Design review of the part built by this model. Coordinates are the model's own, in mm. A direction names the side the tool comes from. Round coordinates to 2 decimals unless told otherwise and drop trailing zeros. Order: outer loops, then holes, each group sorted by start corner. A loop starts at its lowest first (then second) coordinate and runs counter-clockwise, first axis right, second up. Notation, with made-up numbers: (84, 72) - (116, 72) arc R22 ccw to (116, 79) - close; hole circle Ø3 at (36.5, 59.5). An arc over 180 degrees is marked (long way). Use CSV: the item, a comma, the result in double quotes. Start each with the question number.
from build123d import *

# Parameters (mm, degrees)
BASEHEAD_DEPTH = 19.05
HEADFILLET_R   = 1.524


with BuildPart() as part:
    # Sketch1 → BaseHead (new, symmetric)
    with BuildSketch(Plane.XY):
        Polygon((0, -19.05), (0, 19.05), (19.8374, 19.05), (13.495821211, -19.05), align=None)
    extrude(amount=BASEHEAD_DEPTH, both=True)

    # BodySke → Body (revolve)
    with BuildSketch(Plane.XY, mode=Mode.PRIVATE) as body_sk:
        Polygon((0, 0), (0, 12.7), (90.976850605, 12.7), (92.866610605, 10.81024), (92.866610605, 0), align=None)
    revolve(body_sk.sketch.rotate(Axis((0, 0, 0), (1, 0, 0)), 90), axis=Axis((0, 0, 0), (1, 0, 0)))

    # Sketch3 → HeadChamfer (revolve, cut)
    with BuildSketch(Plane(origin=(0, 0, 0), x_dir=(1, 0, 0), z_dir=(0, -0.7071067811865476, 0.7071067811865475))):
        Polygon((0, 19.05), (9.601632975, 39.640768363), (-6.35, 39.640768363), (-6.35, 19.05), align=None)
    revolve(axis=Axis((0, 0, 0), (1, 0, 0)), mode=Mode.SUBTRACT)

    # HeadFillet
    headfillet_edges = [part.edges().sort_by_distance(p)[0] for p in [
        (16.666610593, -7.7e-08, -12.7),
    ]]
    fillet(headfillet_edges, radius=HEADFILLET_R)


solid = part.part
Q1. Tool access review of faces 1 (the cylindrical face through (53.802, -12.592, -1.653)), 2 (the flat face through (10, 0, -19.05)): name each direction out of +Z, -Z, +X, -X, +Y, -Y from which nothing blocks a thin tool from reaching the whole face with its end or side.
Q2. Clearance check with flat-ended pins moving along their axes: pin 1 (1 mm diameter, centred on x = 29, y = 11.5, fed in from -Z); pin 2 (5 mm diameter, centred on x = 65.5, y = -5.5, fed in from +Z); pin 3 (10 mm diameter, centred on x = 69, z = 13, fed in from -Y). State where each tip first meets the part, or that it passes through.
Q3. The part is to be moulded in two halves that separate along Y. For faces 3 (the conical face through (0.894, 14.772, -14.881)), 4 (the flat face through (15.3, -8.2, 13)), 5 (the flat face through (7, -19.05, 0)), say which applies: +Y half, -Y half, draft (parallel to the pull), parting line (faces both ways), or undercut.
Q4. For L1, parallel to Y at x = 62, z = -0.5; L2, parallel to X at y = -14, z = 2.5; L3, parallel to Z at x = 80.5, y = -6, list the stretches that pass through material, from the lowest coordinate up. Write a range as [from, to].
Q5. Take a section at A-A (x = 84). State the section outline as (y, z) points.
Findings below:
1,face 1,"+X"
1,face 2,"-Z, +X, -X, +Y, -Y"
2,pin 1,"stops at z = -6.35"
2,pin 2,"stops at z = 12.34"
2,pin 3,"stops at y = -9.86"
3,face 3,"+Y half"
3,face 4,"undercut"
3,face 5,"-Y half"
4,L1,"y = [-12.69, 12.69]"
4,L2,"x = [0, 14.34]"
4,L3,"z = [-11.19, 11.19]"
5,outline,"circle Ø25.4 at (0, 0)"
